Could you check a few things on this model? Use its own coordinates, in mm. Face numbers are marked on the shaded views. A direction names the side the tool comes from. Give positions to 0.01 mm unless a question says otherwise; leave off trailing zeros. Write each loop counter-clockwise with the first axis right and the second up, starting at its lowest first coordinate (ties: lowest second). Pieces come first, ordered by that corner, then holes. Notation, with made-up numbers: (84.25, 17.5) -> (142.25, 17.5) arc R14 cw to (142.25, 29.5) -> close; hole circle Ø10 at (72.25, -31.5). An arc over 180 degrees is marked (long way). One line per question, with ' | ' between items.
from build123d import *

# Parameters (mm, degrees)
SKETCH1_R                                           = 31
SKETCH1_R_2                                         = 13.384776311
BOSS_EXTRUDE1_DEPTH                                 = 10
CBORE_FOR_M6_HEX_SOCKET_HEAD_CAP_SCREW1_D           = 6.6
CBORE_FOR_M6_HEX_SOCKET_HEAD_CAP_SCREW1_CBORE_D     = 11
CBORE_FOR_M6_HEX_SOCKET_HEAD_CAP_SCREW1_CBORE_DEPTH = 6.4
M3_CLEARANCE_HOLE1_D                                = 3.4
CIRPATTERN1_COUNT                                   = 4


with BuildPart() as part:
    # Sketch1 → Boss-Extrude1 (new body)
    with BuildSketch(Plane(origin=(0, 0, 0), x_dir=(1, 0, 0), z_dir=(0, 1, 0))):
        with Locations(Location((0, 0, 0), (0, 0, 270))):
            Circle(SKETCH1_R)
        with Locations(Location((0, 0, 0), (0, 0, 270))):
            Circle(SKETCH1_R_2, mode=Mode.SUBTRACT)
    extrude(amount=BOSS_EXTRUDE1_DEPTH)

    # CBORE for M6 Hex Socket Head Cap Screw1 (through all)
    with Locations(Plane(origin=(0, 10, 0), x_dir=(1, 0, 0), z_dir=(0, 1, 0))):
        with Locations((0, 25)):
            cbore_for_m6_hex_socket_head_cap_screw1 = CounterBoreHole(CBORE_FOR_M6_HEX_SOCKET_HEAD_CAP_SCREW1_D / 2, CBORE_FOR_M6_HEX_SOCKET_HEAD_CAP_SCREW1_CBORE_D / 2, CBORE_FOR_M6_HEX_SOCKET_HEAD_CAP_SCREW1_CBORE_DEPTH)

    # M3 Clearance Hole1 (through all)
    with Locations(Plane(origin=(0, 10, 0), x_dir=(1, 0, 0), z_dir=(0, 1, 0))):
        with Locations((-13, 13)):
            m3_clearance_hole1 = Hole(M3_CLEARANCE_HOLE1_D / 2)

    # CirPattern1: CBORE for M6 Hex Socket Head Cap Screw1, M3 Clearance Hole1 ×4 about axis
    cirpattern1_axis = Axis((0, 0, 0), (0, 1, 0))
    add([cbore_for_m6_hex_socket_head_cap_screw1.rotate(cirpattern1_axis, i * 360 / CIRPATTERN1_COUNT) for i in range(1, CIRPATTERN1_COUNT)], mode=Mode.SUBTRACT)
    add([m3_clearance_hole1.rotate(cirpattern1_axis, i * 360 / CIRPATTERN1_COUNT) for i in range(1, CIRPATTERN1_COUNT)], mode=Mode.SUBTRACT)


solid = part.part
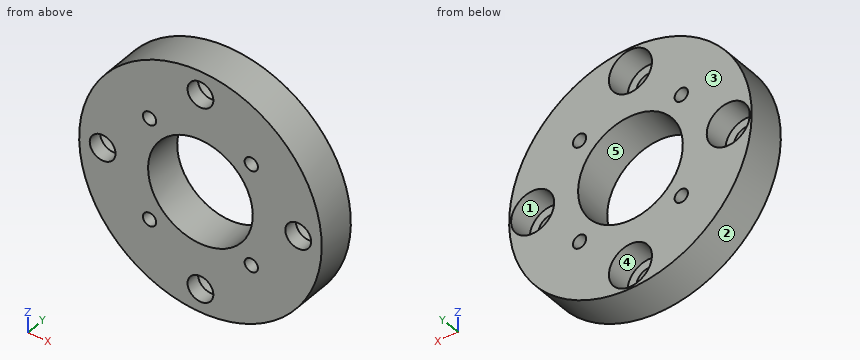
Q1. Imagine slicing it at D-D on x = -25. Please give me the cut outline in (y, z), and give its area (3 significant figures).
Answer below:
outline: (0, -18.33) -> (10, -18.33) -> (10, -5.5) -> (3.6, -5.5) -> (3.6, -3.3) -> (0, -3.3) -> close; (0, 3.3) -> (3.6, 3.3) -> (3.6, 5.5) -> (10, 5.5) -> (10, 18.33) -> (0, 18.33) -> close | area: 272 mm^2
Q2. Imagine slicing it at A-A on z = 0. Please give me the cut outline in (x, y), and give its area (3 significant figures).
Answer below:
outline: (-31, 0) -> (-28.3, 0) -> (-28.3, 3.6) -> (-30.5, 3.6) -> (-30.5, 10) -> (-31, 10) -> close; (-21.7, 0) -> (-13.38, 0) -> (-13.38, 10) -> (-19.5, 10) -> (-19.5, 3.6) -> (-21.7, 3.6) -> close; (13.38, 0) -> (21.7, 0) -> (21.7, 3.6) -> (19.5, 3.6) -> (19.5, 10) -> (13.38, 10) -> close; (28.3, 0) -> (31, 0) -> (31, 10) -> (30.5, 10) -> (30.5, 3.6) -> (28.3, 3.6) -> close | area: 164 mm^2
Q3. Imagine slicing it at C-C on x = 0. Please give me the cut outline in (y, z), and give its area (3 significant figures).
Answer below:
outline: (0, -31) -> (10, -31) -> (10, -30.5) -> (3.6, -30.5) -> (3.6, -28.3) -> (0, -28.3) -> close; (0, -21.7) -> (3.6, -21.7) -> (3.6, -19.5) -> (10, -19.5) -> (10, -13.38) -> (0, -13.38) -> close; (0, 13.38) -> (10, 13.38) -> (10, 19.5) -> (3.6, 19.5) -> (3.6, 21.7) -> (0, 21.7) -> close; (0, 28.3) -> (3.6, 28.3) -> (3.6, 30.5) -> (10, 30.5) -> (10, 31) -> (0, 31) -> close | area: 164 mm^2
Q4. Will these pins go through, and if not, where does the flat tip stop? pin 1 (5.5 mm diameter, centred on x = -2, z = 25, fed in from +Y); pin 2 (2 mm diameter, centred on x = -5.5, y = 5.5, fed in from -Z); pin 3 (2 mm diameter, centred on y = 5.5, z = 21.5, fed in from +X).
Answer below:
pin 1: stops at y = 3.6 | pin 2: stops at z = -30.67 | pin 3: stops at x = 23.25
Q5. On a 3-axis mill with a long thin cutter (end or side, diameter ignored), from which of +Z, -Z, +X, -X, +Y, -Y can I reach the whole of each face in a straight line? I mean the marked faces 4 and 5. Say none if no direction works.
Answer below:
face 4: +Y | face 5: +Y, -Y
Q6. Imagine slicing it at B-B on y = 1.5. Count the separate pieces of the cut face and the enclosed holes in it, and give its area (3 significant figures).
Answer below:
separate pieces: 1 | enclosed holes: 9 | area: 2,280 mm^2
Q7. If I drill on line 1 along X through (y, z) = (0.9, 0); line 2 along X through (y, z) = (3, 14.5), over which ranges is the centre line in solid material (lowest first)?
Answer below:
line 1: x = -31 to -28.3, -21.7 to -13.38, 13.38 to 21.7, 28.3 to 31 | line 2: x = -27.4 to -13.8, -12.2 to 12.2, 13.8 to 27.4
Q8. If we mould it in two halves opening along Z, with no side actions, what happens to the marked faces 1, 2 and 3? For each: +Z half, -Z half, draft (parallel to the pull), parting line (faces both ways), or undercut.
Answer below:
face 1: undercut | face 2: parting line | face 3: draft
